Verification items for the finished model (mm, model axes). A direction names the side the tool comes from. Give positions to 0.01 mm unless a question says otherwise; leave off trailing zeros. Order: outer loops, then holes, each group sorted by start corner. A loop starts at its lowest first (then second) coordinate and runs counter-clockwise, first axis right, second up. Notation, with made-up numbers: (-28, -4.5) -> (-24, -4.5) arc R15 ccw to (-24, 2.5) -> close; hole circle Ø10 at (51.25, 75.5). An arc over 180 degrees is marked (long way). Write each question's results on one line, items separated by ' | '. Start each with the question number.
1. Material ranges on L1, parallel to Y at x = 0, z = 1.9; L2, parallel to Y at x = 4.25, z = 3.3; L3, parallel to X at y = -0.5, z = 0.25 (3 decimals), recorded low to high. Write a range as from..to.
2. Mould release check, pull along X, two halves, no side actions. Record for faces 4 (the face through (-14, 0, 2)), 5 (the face through (3, 0, 0)): +X half, -X half, draft (parallel to the pull), parting line (faces both ways), or undercut.
3. Cross-section at B-B, the plane z = 0.9. Enter the section's corners in (x, y) (3 decimals), then the cut area to 3 significant figures.
4. Cross-section at A-A, the plane x = 0. Enter the section's corners in (y, z) (3 decimals).
5. Depth check by flat-ended pin: pin 1 Ø1.5 at (y, z) = (10.5, 2) entering from +X; pin 2 Ø3.5 at (x, y) = (-5.75, 5.75) entering from +Z; pin 3 Ø2 at (x, z) = (0, 2) entering from -Y. Enter the tip coordinate at first touch or a pass-through.
6. Set-up check for faces 1 (the face through (8, 5, 3)), 2 (the face through (-1.685, -8, 1)), 3 (the face through (3.1, -7.2, 2.6)): record each of +Z, -Z, +X, -X, +Y, -Y from which the full face is reachable in a straight line by a thin tool's end or side.
7. Cross-section at C-C, the plane x = 7.75. Enter the section's corners in (y, z), then the cut area to 3 significant figures.
from build123d import *

# Parameters (mm, degrees)
F1_DEPTH = 1.5
F0_R     = 3
F0_R_2   = 1.575
F2_DEPTH = 4.5
F0_R_3   = 1.625
F3_DEPTH = 3


# Not quite as in the source:
# - a feature names something its author has since deleted; it is built from what else it names


with BuildPart() as f1:
    # F0 (on Top) → F1 (new body)
    with BuildSketch(Plane.XY):
        with BuildLine():
            Line((-1.685, -4.7075232341), (-1.685, -2.6020712903))
            ThreePointArc((-1.685, -2.6020712903), (-2.7233710728, -1.4809625248), (-3.1, 0))
            Line((-3.1, 0), (-3.1, -3.9230090492))
            ThreePointArc((-3.1, -3.9230090492), (-2.4244425909, -4.3728798432), (-1.685, -4.7075232341))
        make_face()
        with BuildLine():
            Line((-1.685, -14.905058705), (-1.685, -4.7075232341))
            ThreePointArc((-1.685, -4.7075232341), (-2.4244425909, -4.3728798432), (-3.1, -3.9230090492))
            Line((-3.1, -3.9230090492), (-3.1, -14.6761711628))
            ThreePointArc((-3.1, -14.6761711628), (-2.3952356099, -14.8075266798), (-1.685, -14.905058705))
        make_face()
        with BuildLine():
            ThreePointArc((3.1, -3.9230090492), (2.4244425909, -4.3728798432), (1.685, -4.7075232341))
            Line((1.685, -4.7075232341), (1.685, -14.905058705))
            ThreePointArc((1.685, -14.905058705), (2.3952356099, -14.8075266798), (3.1, -14.6761711628))
            Line((3.1, -14.6761711628), (3.1, -7.1604074647))
            ThreePointArc((3.1, -7.1604074647), (2.7452425971, -5.7452425971), (3.1, -4.3300777296))
            Line((3.1, -4.3300777296), (3.1, -3.9230090492))
        make_face()
        with BuildLine():
            ThreePointArc((-1.685, 0), (0, 1.685), (1.685, 0))
            Line((1.685, 0), (1.685, -2.6020712903))
            ThreePointArc((1.685, -2.6020712903), (2.7233710728, -1.4809625248), (3.1, 0))
            ThreePointArc((3.1, 0), (0, 3.1), (-3.1, 0))
            ThreePointArc((-3.1, 0), (-2.7233710728, -1.4809625248), (-1.685, -2.6020712903))
            Line((-1.685, -2.6020712903), (-1.685, 0))
        make_face()
        with BuildLine():
            ThreePointArc((-3.1, 0), (0, 3.1), (3.1, 0))
            Line((3.1, 0), (3.1, -3.9230090492))
            ThreePointArc((3.1, -3.9230090492), (4.5, -2.1794494718), (5, 0))
            ThreePointArc((5, 0), (-2.1794494718, 4.5), (-3.1, -3.9230090492))
            Line((-3.1, -3.9230090492), (-3.1, 0))
        make_face()
        with BuildLine():
            ThreePointArc((3.1, 0), (2.7233710728, -1.4809625248), (1.685, -2.6020712903))
            Line((1.685, -2.6020712903), (1.685, -4.7075232341))
            ThreePointArc((1.685, -4.7075232341), (2.4244425909, -4.3728798432), (3.1, -3.9230090492))
            Line((3.1, -3.9230090492), (3.1, 0))
        make_face()
        with BuildLine():
            Line((3.1, -7.1604074647), (3.1, -4.3300777296))
            ThreePointArc((3.1, -4.3300777296), (2.7452425971, -5.7452425971), (3.1, -7.1604074647))
        make_face()
    extrude(amount=F1_DEPTH)

    # F0 (on Top) → F2 (join)
    with BuildSketch(Plane.XY):
        with BuildLine():
            ThreePointArc((-3.1, 0), (0, 3.1), (3.1, 0))
            Line((3.1, 0), (3.1, -3.9230090492))
            ThreePointArc((3.1, -3.9230090492), (4.5, -2.1794494718), (5, 0))
            ThreePointArc((5, 0), (-2.1794494718, 4.5), (-3.1, -3.9230090492))
            Line((-3.1, -3.9230090492), (-3.1, 0))
        make_face()
        with BuildLine():
            ThreePointArc((5, 0), (4.5, -2.1794494718), (3.1, -3.9230090492))
            Line((3.1, -3.9230090492), (3.1, -4.3300777296))
            ThreePointArc((3.1, -4.3300777296), (6.4747191933, -2.8352831652), (8.7452425971, -5.7452425971))
            ThreePointArc((8.7452425971, -5.7452425971), (6.4747191933, -8.6552020291), (3.1, -7.1604074647))
            Line((3.1, -7.1604074647), (3.1, -14.6761711628))
            ThreePointArc((3.1, -14.6761711628), (11.6511801977, -9.4472218138), (15, 0))
            ThreePointArc((15, 0), (-9.4472218138, 11.6511801977), (-3.1, -14.6761711628))
            Line((-3.1, -14.6761711628), (-3.1, -3.9230090492))
            ThreePointArc((-3.1, -3.9230090492), (-2.1794494718, 4.5), (5, 0))
        make_face()
        with Locations((-6.7175144213, -6.7175144213)):
            Circle(F0_R, mode=Mode.SUBTRACT)
        with Locations((-12.425, 0)):
            Circle(F0_R_2, mode=Mode.SUBTRACT)
        with Locations((-5.7452425971, 5.7452425971)):
            Circle(F0_R, mode=Mode.SUBTRACT)
        with Locations((6.7175144213, 6.7175144213)):
            Circle(F0_R, mode=Mode.SUBTRACT)
        with Locations((12.425, 0)):
            Circle(F0_R_2, mode=Mode.SUBTRACT)
        with Locations((0, 12.425)):
            Circle(F0_R_2, mode=Mode.SUBTRACT)
    extrude(amount=F2_DEPTH)

    # F0 (on Top) → F3 (join)
    with BuildSketch(Plane.XY):
        with Locations((-5.7452425971, 5.7452425971)):
            Circle(F0_R)
        with Locations((-5.7452425971, 5.7452425971)):
            Circle(F0_R_2, mode=Mode.SUBTRACT)
        with Locations((6.7175144213, 6.7175144213)):
            Circle(F0_R)
        with Locations((6.7175144213, 6.7175144213)):
            Circle(F0_R_3, mode=Mode.SUBTRACT)
        with BuildLine():
            ThreePointArc((8.7452425971, -5.7452425971), (6.4747191933, -2.8352831652), (3.1, -4.3300777296))
            Line((3.1, -4.3300777296), (3.1, -7.1604074647))
            ThreePointArc((3.1, -7.1604074647), (6.4747191933, -8.6552020291), (8.7452425971, -5.7452425971))
        make_face()
        with Locations((5.7452425971, -5.7452425971)):
            Circle(F0_R_2, mode=Mode.SUBTRACT)
        with Locations((-6.7175144213, -6.7175144213)):
            Circle(F0_R)
        with Locations((-6.7175144213, -6.7175144213)):
            Circle(F0_R_3, mode=Mode.SUBTRACT)
    extrude(amount=F3_DEPTH)


solid = f1.part
Results below:
1) L1: y = 3.1..10.85, 14..15 | L2: y = -14.39..-8.35, -3.14..5.01, 8.42..14.39 | L3: x = -14.992..-13.919, -10.931..-1.685, 1.685..10.931, 13.919..14.992
2) face 4: undercut | face 5: draft
3) outline: (-1.685, -14.905) -> (-1.685, 0) arc R1.685 cw to (1.685, 0) -> (1.685, -14.905) arc R15 ccw (long way) to start; hole circle Ø3.15 at (-12.425, 0); hole circle Ø3.25 at (-6.718, -6.718); hole circle Ø3.15 at (-5.745, 5.745); hole circle Ø3.15 at (0, 12.425); hole circle Ø3.15 at (5.745, -5.745); hole circle Ø3.25 at (6.718, 6.718); hole circle Ø3.15 at (12.425, 0) | area: 596 mm²
4) outline: (1.685, 0) -> (10.85, 0) -> (10.85, 4.5) -> (3.1, 4.5) -> (3.1, 1.5) -> (1.685, 1.5) -> close; (14, 0) -> (15, 0) -> (15, 4.5) -> (14, 4.5) -> close
5) pin 1: stops at x = 11.4 | pin 2: stops at z = 3 | pin 3: stops at y = 1.45
6) face 1: +Z | face 2: +Z, -Z, -Y | face 3: +Z, -Y
7) outline: (-12.84, 0) -> (5.46, 0) -> (5.46, 3) -> (3.9, 3) -> (3.9, 4.5) -> (-3.51, 4.5) -> (-3.51, 3) -> (-7.98, 3) -> (-7.98, 4.5) -> (-12.84, 4.5) -> close; (7.97, 0) -> (12.84, 0) -> (12.84, 4.5) -> (9.53, 4.5) -> (9.53, 3) -> (7.97, 3) -> close | area: 92.9 mm²
